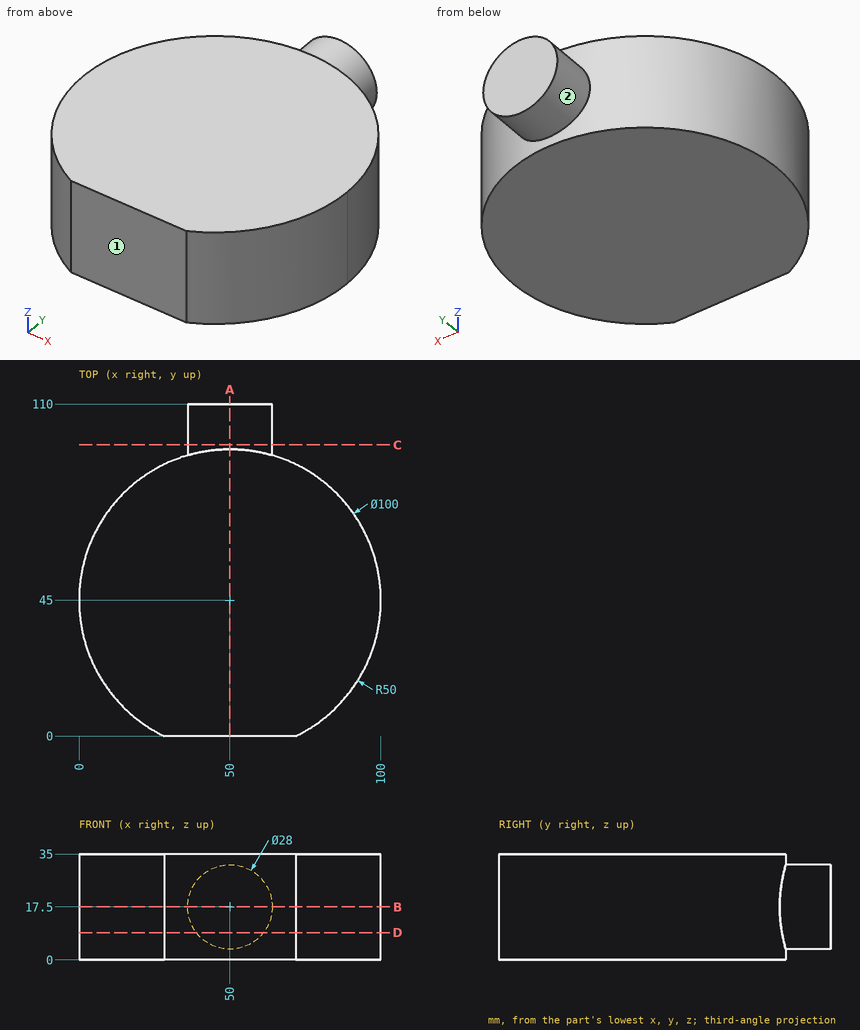
Input: dimensioned drawing with shaded views. Units: mm. Origin: part minimum x, y, z. A direction names the side the tool comes from. Coordinates: 2 decimals unless noted, no trailing zeros. Order: outer loops, then holes, each group sorted by start corner. A loop starts at its lowest first (then second) coordinate and runs counter-clockwise, first axis right, second up.
1. Cut plane B-B, the plane z = 17.5. Return loops of the section in (x, y), plus the area to 3 significant figures.
Checked values:
outline: (28.21, 0) - (71.79, 0) arc R50 ccw to (64, 93) - (64, 110) - (36, 110) - (36, 93) arc R50 ccw to start
area: 8,150 mm2
2. Cut plane D-D, the plane z = 9. Return loops of the section in (x, y), plus the area to 3 significant figures.
Checked values:
outline: (28.21, 0) - (71.79, 0) arc R50 ccw to (61.12, 93.75) - (61.12, 110) - (38.88, 110) - (38.88, 93.75) arc R50 ccw to start
area: 8,050 mm2
3. Cut plane C-C, the plane y = 96.5. Return loops of the section in (x, z).
Checked values:
outline: circle Ø28 at (50, 17.5)
4. Access query for the marked faces 1 and 2. Directions: +Z, -Z, +X, -X, +Y, -Y. A direction counts if a zero-diameter tool reaches every point of the face in a straight line with its end or side. Return the directions, or none.
Checked values:
face 1: +Z, -Z, +X, -X, -Y
face 2: +Y
5. Contact query for flat-ended pins moving along their axis: P1, Ø3, axis at x = 25, z = 25, coming from the +Y side; P2, Ø1, axis at y = 68, z = 22.5, coming from the -X side; P3, Ø3, axis at x = 65.5, z = 10, coming from the +Y side. Output: stop coordinate, or through.
Checked values:
P1: stops at y = 89.13
P2: stops at x = 5.35
P3: stops at y = 93
6. Ray query, line 1 along X through (y, z) = (86, 28.5); line 2 along X through (y, z) = (38, 24); line 3 along Y through (x, z) = (68, 3). Return the intervals inside material, ascending.
Checked values:
line 1: x = 21.38 to 78.62
line 2: x = 0.49 to 99.51
line 3: y = 0 to 91.65
7. Cut plane A-A, the plane x = 50. Return loops of the section in (y, z), plus the area to 4 significant figures.
Checked values:
outline: (0, 0) - (95, 0) - (95, 3.5) - (110, 3.5) - (110, 31.5) - (95, 31.5) - (95, 35) - (0, 35) - close
area: 3,745 mm2
